Geometry: final body of the model. Coordinates: model frame, mm. Face numbers are marked on the shaded views. A direction names the side the tool comes from. Give positions to 0.01 mm unless a question says otherwise; leave off trailing zeros. Write each loop counter-clockwise with the first axis right and the second up, starting at its lowest first coordinate (ties: lowest second). Pieces come first, ordered by that corner, then holes. Notation, with made-up numbers: (47.25, 36.25) -> (73.25, 36.25) arc R32 cw to (73.25, 64.25) -> close; hole circle Ø4 at (35.5, 23). An arc over 180 degrees is marked (long way). Answer in a Markdown table with one row per item. Add a question column.
Item 1: Draft query along Y for the marked faces 1, 2 and 3. Return one class per face: +Y half, -Y half, draft (parallel to the pull), parting line (faces both ways), or undercut.
Item 2: Material intervals for probe 1 along X at (y, z) = (-30, 2.75); probe 2 along Y at (x, z) = (1, 1.15); probe 3 along X at (y, z) = (-32, 4.1), sorted ascending. Write a range as from..to.
Item 3: Section query A-A on z = 1.4. Output: boundary loops of the cut face in (x, y).
Item 4: Section query D-D on y = 36.5. Output: boundary loops of the cut face in (x, z).
Item 5: Access query for the marked faces 4 and 5. Directions: +Z, -Z, +X, -X, +Y, -Y. A direction counts if a zero-diameter tool reaches every point of the face in a straight line with its end or side. Return the directions, or none.
Item 6: First-contact query: P1, Ø1, axis at x = -11.5, z = 5, coming from the -Y side. Flat tip, straight axial feed; report the tip coordinate or a pass-through.
Item 7: Section query B-B on y = -32. Output: boundary loops of the cut face in (x, z), plus the area to 3 significant figures.
Item 8: Section query C-C on x = 1.5. Output: boundary loops of the cut face in (y, z).
```python
from build123d import *

# Parameters (mm, degrees)
F0_R     = 4
F1_DEPTH = 6


with BuildPart() as f1:
    # F0 (on Top) → F1 (new body)
    with BuildSketch(Plane.XY):
        with BuildLine():
            Line((-8, 50), (-15, 50))
            Line((-15, 50), (-15, -45))
            ThreePointArc((-15, -45), (-13.535534, -48.535534), (-10, -50))
            Line((-10, -50), (0, -50))
            Line((0, -50), (10, -50))
            ThreePointArc((10, -50), (13.535534, -48.535534), (15, -45))
            Line((15, -45), (15, 50))
            Line((15, 50), (8, 50))
            Line((8, 50), (4.946622, 29.271351))
            ThreePointArc((4.946622, 29.271351), (0, 25), (-4.946622, 29.271351))
            Line((-4.946622, 29.271351), (-8, 50))
        make_face()
        with BuildLine():
            ThreePointArc((3, -30), (2.12132, -32.12132), (0, -33))
            ThreePointArc((0, -33), (-2.12132, -27.87868), (3, -30))
        make_face(mode=Mode.SUBTRACT)
        Circle(F0_R, mode=Mode.SUBTRACT)
    extrude(amount=F1_DEPTH)


solid = f1.part
```
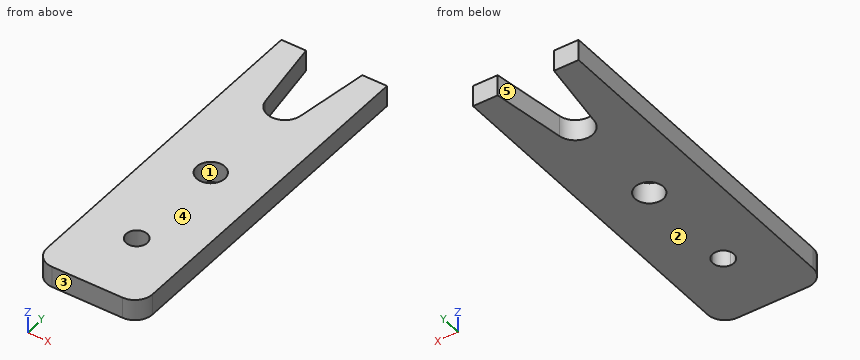
Findings below:
| question | item | result |
|---|---|---|
| 1 | face 1 | undercut |
| 1 | face 2 | draft |
| 1 | face 3 | -Y half |
| 2 | probe 1 | x = -15..-3, 3..15 |
| 2 | probe 2 | y = -50..-32.83, -27.17..-3.87, 3.87..25.1 |
| 2 | probe 3 | x = -15..-2.24, 2.24..15 |
| 3 | outline | (-15, -45) arc R5 ccw to (-10, -50) -> (10, -50) arc R5 ccw to (15, -45) -> (15, 50) -> (8, 50) -> (4.95, 29.27) arc R5 cw to (-4.95, 29.27) -> (-8, 50) -> (-15, 50) -> close; hole circle Ø8 at (0, 0); hole (0, -33) arc R3 ccw to (3, -30) arc R3 ccw (long way) to start |
| 4 | outline | (-15, 0) -> (-6.01, 0) -> (-6.01, 6) -> (-15, 6) -> close; (6.01, 0) -> (15, 0) -> (15, 6) -> (6.01, 6) -> close |
| 5 | face 4 | +Z, +X, -X, +Y, -Y |
| 5 | face 5 | +Z, -Z, +Y |
| 6 | P1 | stops at y = -49.9 |
| 7 | outline | (-15, 0) -> (-2.24, 0) -> (-2.24, 6) -> (-15, 6) -> close; (2.24, 0) -> (15, 0) -> (15, 6) -> (2.24, 6) -> close |
| 7 | area | 153 mm^2 |
| 8 | outline | (-50, 0) -> (-32.6, 0) -> (-32.6, 6) -> (-50, 6) -> close; (-27.4, 0) -> (-3.71, 0) -> (-3.71, 6) -> (-27.4, 6) -> close; (3.71, 0) -> (25.23, 0) -> (25.23, 6) -> (3.71, 6) -> close |
